Could you check a few things on this model? Use its own coordinates, in mm. Face numbers are marked on the shaded views. A direction names the side the tool comes from. Give positions to 0.01 mm unless a question says otherwise; leave off trailing zeros. Loops run counter-clockwise (first coordinate to the right, second up) from the corner with the lowest first, then second, coordinate; pieces in that order, holes last. Notation, with made-up numbers: M -7,41 L 6,41 A15 ccw 6,63 Z; hole C -11,34 d6. An arc over 180 degrees is marked long. Return JSON: item names as keys, results as strings. Group by question number.
1. If we section it at A-A (z = -6.5): Write out the boundary of the cut face in (x, y), plus the area to 3 significant figures.
2. For pin 1 (10 mm diameter, centred on y = 5.5, z = -8.5, fed in from -X); pin 2 (10 mm diameter, centred on y = 5, z = -4.5, fed in from -X), each with a flat end and sliding along its axis, tell me the tip position at first contact or that it passes through.
3. If we section it at C-C (x = -118): Write out the boundary of the cut face in (y, z), plus the area to 3 significant figures.
4. Please list where this line runs through material, in increasing order: line 1 (Z direction, x = -127, y = -6.5).
5. If we mould it in two halves opening along Y, with no side actions, what happens to the marked faces 3, 4 and 5? For each: +Y half, -Y half, draft (parallel to the pull), parting line (faces both ways), or undercut.
6. For the marked faces 1 and 2, which set-ups out of +Z, -Z, +X, -X, +Y, -Y let a thin tool reach every point of the face, with its end or its side?
7. If we section it at D-D (y = -4): Write out the boundary of the cut face in (x, z).
8. If we section it at B-B (y = 4.5): Write out the boundary of the cut face in (x, z), plus the area to 4 significant figures.
```python
from build123d import *

# Parameters (mm, degrees)
SKETCH3_W           = 25.4
SKETCH3_H           = 25.4
SKETCH3_W_2         = 19.304
SKETCH3_H_2         = 19.304
BOSS_EXTRUDE1_DEPTH = 154.14
FILLET1_R           = 2.5
FILLET2_R           = 1
CUT_EXTRUDE2_DEPTH  = 157.734136677


with BuildPart() as part:
    # Sketch3 → Boss-Extrude1 (new body)
    with BuildSketch(Plane(origin=(0, 0, 0), x_dir=(0, 0, -1), z_dir=(1, 0, 0))):
        Rectangle(SKETCH3_W, SKETCH3_H)
        Rectangle(SKETCH3_W_2, SKETCH3_H_2, mode=Mode.SUBTRACT)
    extrude(amount=-BOSS_EXTRUDE1_DEPTH)

    # Fillet1
    fillet1_edges = [part.edges().sort_by_distance(p)[0] for p in [
        (-77.07, -12.7, -12.7),
        (-77.07, -12.7, 12.7),
        (-77.07, 12.7, 12.7),
        (-77.07, 12.7, -12.7),
    ]]
    fillet(fillet1_edges, radius=FILLET1_R)

    # Fillet2
    fillet2_edges = [part.edges().sort_by_distance(p)[0] for p in [
        (-77.07, 9.652, -9.652),
        (-77.07, -9.652, -9.652),
        (-77.07, -9.652, 9.652),
        (-77.07, 9.652, 9.652),
    ]]
    fillet(fillet2_edges, radius=FILLET2_R)

    # Sketch5 → Cut-Extrude2 (cut, through all)
    with BuildSketch(Plane(origin=(0, 0, -12.7), x_dir=(-1, 0, 0), z_dir=(0, 0, -1))):
        Polygon((0, 10.2), (7.440661044, 10.2), (8.252960284, 12.7), (0, 12.7), align=None)
        Polygon((0.812299241, -10.2), (7.440661044, 10.2), (0, 10.2), (0, -10.2), align=None)
        Polygon((0, -12.7), (0.812299241, -10.2), (0, -10.2), align=None)
        Polygon((154.14, 10.2), (146.699338956, 10.2), (153.327700759, -10.2), (154.14, -10.2), align=None)
        Polygon((154.14, -10.2), (153.327700759, -10.2), (154.14, -12.7), align=None)
        Polygon((154.14, 12.7), (145.887039716, 12.7), (146.699338956, 10.2), (154.14, 10.2), align=None)
    extrude(amount=-CUT_EXTRUDE2_DEPTH, mode=Mode.SUBTRACT)


solid = part.part
```
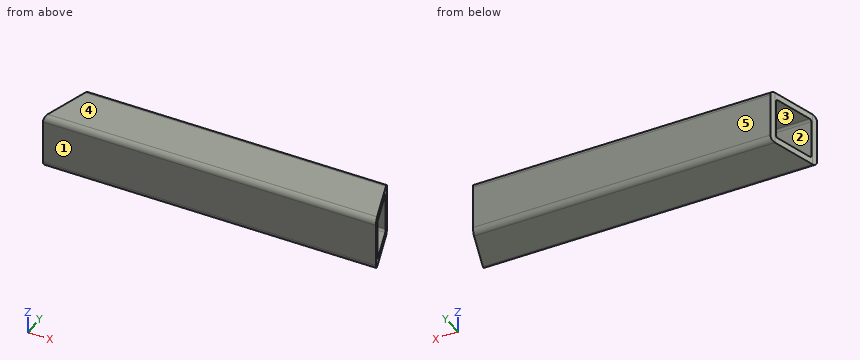
Answer:
{
 "1": {"outline": "M -154.14,-12.7 L 0,-12.7 L -0.99,-9.65 L -153.15,-9.65 Z; M -146.88,9.65 L -7.26,9.65 L -8.25,12.7 L -145.89,12.7 Z", "area": "889 mm²"},
 "2": {"pin 1": "stops at x = -149.81", "pin 2": "stops at x = -146.88"},
 "3": {"outline": "M -12.7,-10.2 A2.5 ccw -10.2,-12.7 L 10.2,-12.7 A2.5 ccw 12.7,-10.2 L 12.7,10.2 A2.5 ccw 10.2,12.7 L -10.2,12.7 A2.5 ccw -12.7,10.2 Z; hole M -9.65,-8.65 A1 ccw -8.65,-9.65 L 8.65,-9.65 A1 ccw 9.65,-8.65 L 9.65,8.65 A1 ccw 8.65,9.65 L -8.65,9.65 A1 ccw -9.65,8.65 Z", "area": "268 mm²"},
 "4": {"line 1": "z = -12.7 to -9.65, 9.65 to 12.7"},
 "5": {"face 3": "undercut", "face 4": "draft", "face 5": "+Y half"},
 "6": {"face 1": "+Z, -Z, +X, -X, -Y", "face 2": "+X, -X"},
 "7": {"outline": "M -151.31,-12.7 L -2.83,-12.7 L -2.83,-9.65 L -151.31,-9.65 Z; M -151.31,9.65 L -2.83,9.65 L -2.83,12.7 L -151.31,12.7 Z"},
 "8": {"outline": "M -148.55,-12.7 L -5.59,-12.7 L -5.59,-9.65 L -148.55,-9.65 Z; M -148.55,9.65 L -5.59,9.65 L -5.59,12.7 L -148.55,12.7 Z", "area": "871.5 mm²"}
}
